Check sheet for the modelled part. Datum: model origin and axes. Units: mm. Face numbers are marked on the shaded views. A direction names the side the tool comes from. Round coordinates to 2 decimals unless told otherwise and drop trailing zeros. Loops run counter-clockwise (first coordinate to the right, second up) from the corner with the lowest first, then second, coordinate; pieces in that order, holes last. Notation, with made-up numbers: (25, -3) - (72, -3) arc R29 cw to (72, 28) - close; hole circle Ø3 at (39, -34). An arc over 180 degrees is marked (long way). Put each result on its own line as item: value. Start each with the question number.
Item 1: Material ranges on line 1 along X through (y, z) = (19.75, -12.7) (3 decimals); line 2 along X through (y, z) = (17, -12); line 3 along X through (y, z) = (24.75, -63.5) (3 decimals), recorded low to high.
Item 2: Section check A-A, the plane y = 12. Record the cut outline in (x, z) (3 decimals), and give its area (3 significant figures).
Item 3: Section check C-C, the plane x = 219. Record the cut outline in (y, z).
Item 4: Gauge pin test, flat ends, axial feed: pin 1 Ø1.5 at (x, z) = (435, -26.5) entering from +Y; pin 2 Ø14 at (y, z) = (12, -63) entering from -X; pin 3 Ø6 at (x, y) = (321.5, 15.5) entering from -Z; pin 4 Ø7 at (y, z) = (26.5, -36.5) entering from -X. Record the tip position at first contact, or that the pin passes through.
Item 5: Tool access check on the marked faces 1, 2, 3 and 4. Record the directions out of +Z, -Z, +X, -X, +Y, -Y that give a thin tool (end or side, any length) a straight path to the whole face; none if there is none.
Item 6: Section check B-B, the plane z = -33. Record the cut outline in (x, y).
from build123d import *

# Parameters (mm, degrees)
SKETCH2_R           = 6.35
SKETCH2_R_2         = 3.175
BOSS_EXTRUDE1_DEPTH = 25.4
SKETCH12_W          = 38.1
SKETCH12_H          = 25.4
SKETCH12_H_2        = 2.54
BOSS_EXTRUDE2_DEPTH = 25.4
BOSS_EXTRUDE3_DEPTH = 50.8
SKETCH14_R          = 3.175
CUT_EXTRUDE1_DEPTH  = 39.624
FILLET1_R           = 7.62


with BuildPart() as part:
    # Sketch2 → Boss-Extrude1 (new body)
    with BuildSketch(Plane(origin=(0, 0, 0), x_dir=(1, 0, 0), z_dir=(0, 1, 0))):
        with BuildLine():
            ThreePointArc((0, 25.4), (-12.7, 12.7), (0, 0))
            Line((0, 0), (565.15, 0))
            ThreePointArc((565.15, 0), (577.85, 12.7), (565.15, 25.4))
            Line((565.15, 25.4), (0, 25.4))
        make_face()
        with Locations(Location((0, 12.7, 0), (0, 0, 270))):
            Circle(SKETCH2_R, mode=Mode.SUBTRACT)
        with Locations(Location((120.65, 12.7, 0), (0, 0, 270))):
            Circle(SKETCH2_R_2, mode=Mode.SUBTRACT)
        with Locations(Location((565.15, 12.7, 0), (0, 0, 270))):
            Circle(SKETCH2_R, mode=Mode.SUBTRACT)
    extrude(amount=BOSS_EXTRUDE1_DEPTH)

    # Sketch12 → Boss-Extrude2 (add)
    with BuildSketch(Plane(origin=(0, 0, -25.4), x_dir=(-1, 0, 0), z_dir=(0, 0, -1))):
        with Locations((-406.4, 12.7)):
            Rectangle(SKETCH12_W, SKETCH12_H)
        with Locations((-406.4, -1.27)):
            Rectangle(SKETCH12_W, SKETCH12_H_2)
        with Locations((-406.4, 26.67)):
            Rectangle(SKETCH12_W, SKETCH12_H_2)
    extrude(amount=-BOSS_EXTRUDE2_DEPTH)

    # Sketch13 → Boss-Extrude3 (add)
    with BuildSketch(Plane(origin=(0, 0, -25.4), x_dir=(-1, 0, 0), z_dir=(0, 0, -1))):
        Polygon((-387.35, 27.94), (-425.45, 27.94), (-425.45, 25.4), (-425.45, 0), (-425.45, -2.54), (-387.35, -2.54), (-387.35, 0), (-387.35, 3.81), (-419.1, 3.81), (-419.1, 21.59), (-387.35, 21.59), (-387.35, 25.4), align=None)
    extrude(amount=BOSS_EXTRUDE3_DEPTH)

    # Sketch14 → Cut-Extrude1 (cut, symmetric)
    with BuildSketch(Plane.XZ.offset(-21.59)):
        with Locations(Location((393.7, -63.5, 0), (0, 0, 90))):
            Circle(SKETCH14_R)
    extrude(amount=CUT_EXTRUDE1_DEPTH, both=True, mode=Mode.SUBTRACT)

    # Fillet1
    fillet1_edges = [part.edges().sort_by_distance(p)[0] for p in [
        (387.35, 24.765, -76.2),
        (387.35, 0.635, -76.2),
    ]]
    fillet(fillet1_edges, radius=FILLET1_R)


solid = part.part
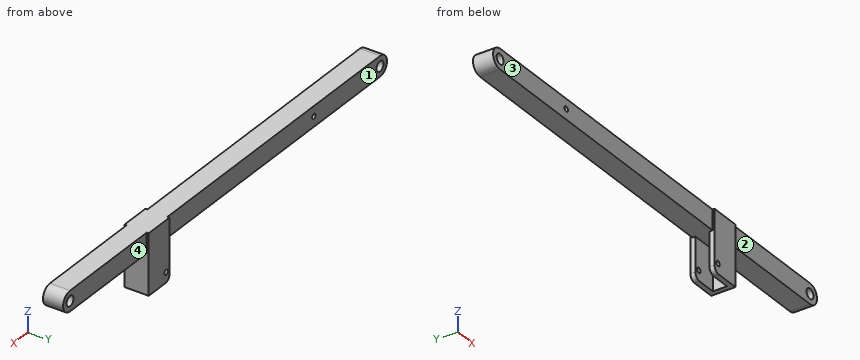
Check result:
1. line 1: -12.7 to -6.35, 6.35 to 117.475, 123.825 to 558.8, 571.5 to 577.85
1. line 2: -12.68 to -6.31, 6.31 to 117.55, 123.75 to 558.84, 571.46 to 577.83
1. line 3: 387.35 to 390.525, 396.875 to 425.45
2. outline: (0, -25.4) - (419.1, -25.4) - (419.1, -76.2) - (425.45, -76.2) - (425.45, -25.4) - (565.15, -25.4) arc R12.7 ccw to (565.15, 0) - (0, 0) arc R12.7 ccw to start; hole circle Ø12.7 at (0, -12.7); hole circle Ø6.35 at (120.65, -12.7); hole circle Ø12.7 at (565.15, -12.7)
2. area: 14,900 mm²
3. outline: (0, -25.4) - (25.4, -25.4) - (25.4, 0) - (0, 0) - close
4. pin 1: through
4. pin 2: x = 419.1
4. pin 3: z = -25.4
4. pin 4: x = 387.35
5. face 1: +Z, -Z, -X, +Y
5. face 2: +Z, -Z, +X, -Y
5. face 3: +Z, -Z, -X, -Y
5. face 4: +Z, -Z, +X, +Y
6. outline: (387.35, -2.54) - (425.45, -2.54) - (425.45, 27.94) - (387.35, 27.94) - (387.35, 21.59) - (419.1, 21.59) - (419.1, 3.81) - (387.35, 3.81) - close
